The model under review builds one solid part; all positions refer to its coordinate system, in mm. A direction names the side the tool comes from. Coordinates: 2 decimals unless noted, no trailing zeros. Order: outer loops, then holes, each group sorted by start corner. A loop starts at its lowest first (then second) coordinate and runs counter-clockwise, first axis right, second up. Notation, with made-up numbers: (-39.75, 54) -> (-10.75, 54) arc R25 ccw to (-10.75, 68) -> close; hole circle Ø11 at (48, 25.5). An arc over 180 degrees is marked (long way). Use one line per item in the form item = value. Start each with the question number.
(1) Wall thickness on line 1 along X through (y, z) = (-2.4, 19); line 2 along X through (y, z) = (-2.5, -15.25); line 3 along Z through (x, y) = (-9.5, -0.75): over which ranges is each line inside the solid? List them lowest first.
(2) Insertion check: pin 1 Ø1.7 at (x, z) = (14.5, 14) entering from -Y; pin 2 Ø1 at (y, z) = (-1, -61.5) entering from +X. Each pin has a flat end and moves straight along its axis. Give the tip position at first contact, or say it passes through.
(3) Take a section at B-B (z = -50). State the section outline as (x, y) points.
(4) Mouldability with a two-part tool opening along X and no side actions: class faces 1 (the flat face through (-1, 0, -1)), 2 (the cylindrical face through (-39, -1, -50)), 3 (the flat face through (68.84, -1.48, 68.53)) as +X half, -X half, draft (parallel to the pull), parting line (faces both ways), or undercut.
(5) Take a section at C-C (y = -1.5). State how many separate pieces and enclosed holes the cut face has, then the cut area to 3 significant figures.
(6) For faces 4 (the cylindrical face through (-13.324, -2.507, -17.351)), 5 (the cylindrical face through (7, -1, -50)), 6 (the flat face through (-68.84, -1.48, -68.53)), list the 3-axis set-ups (+Z, -Z, +X, -X, +Y, -Y) from which the entire face can be reached by the end or side of a thin tool; tool diameter is ignored.
(7) Take a section at A-A (x = -26.5). State the section outline as (y, z) points, then the cut area to 3 significant figures.
```python
from build123d import *

# Parameters (mm, degrees)
SKETCH1_W                                  = 160
SKETCH1_H                                  = 160
BOSS_EXTRUDE1_DEPTH                        = 3
CUT_EXTRUDE2_REACH                         = 115.177
CUT_EXTRUDE1_REACH                         = 115.177
SKETCH2_R                                  = 2.55
MIRROR2_AT_THE_SECOND_PLANE_COPY_1_REACH   = 115.177
MIRROR2_AT_THE_SECOND_PLANE_COPY_2_REACH   = 115.177
MIRROR2_AT_THE_SECOND_PLANE_COPY_2_SKETC_R = 2.55
CUT_EXTRUDE3_REACH                         = 115.177
SKETCH8_R                                  = 1.525
CUT_EXTRUDE4_REACH                         = 115.177
SKETCH10_R                                 = 2.85
CUT_EXTRUDE6_DEPTH                         = 1


with BuildPart() as part:
    # Sketch1 → Boss-Extrude1 (new body)
    with BuildSketch(Plane(origin=(0, 0, 0), x_dir=(1, 0, 0), z_dir=(0, 1, 0))):
        Rectangle(SKETCH1_W, SKETCH1_H)
    extrude(amount=-BOSS_EXTRUDE1_DEPTH)

    # Sketch6 → Cut-Extrude2 (cut, up to next)
    with BuildSketch(Plane(origin=(0, 0, 0), x_dir=(1, 0, 0), z_dir=(0, 1, 0)), mode=Mode.PRIVATE) as cut_extrude2_sk1:
        Polygon((-80, -57.372583002), (-57.372583002, -80), (-80, -80), align=None)
    cut_extrude2_tool1 = extrude(cut_extrude2_sk1.sketch, amount=-CUT_EXTRUDE2_REACH, mode=Mode.PRIVATE) & part.part
    cut_extrude2 = cut_extrude2_tool1.solids().sort_by_distance((-72.457528, 0, 72.457528))[0]
    add(cut_extrude2, mode=Mode.SUBTRACT)

    # Sketch2 → Cut-Extrude1 (cut, up to next)
    with BuildSketch(Plane(origin=(0, 0, 0), x_dir=(1, 0, 0), z_dir=(0, 1, 0)), mode=Mode.PRIVATE) as cut_extrude1_sk1:
        with Locations(Location((-67.272077939, -55.95836944, 0), (0, 0, 270))):
            Circle(SKETCH2_R)
    cut_extrude1_tool1 = extrude(cut_extrude1_sk1.sketch, amount=-CUT_EXTRUDE1_REACH, mode=Mode.PRIVATE) & part.part
    # Sketch2 → Cut-Extrude1 (cut, up to next)
    with BuildSketch(Plane(origin=(0, 0, 0), x_dir=(1, 0, 0), z_dir=(0, 1, 0)), mode=Mode.PRIVATE) as cut_extrude1_sk2:
        with Locations(Location((-55.95836944, -67.272077939, 0), (0, 0, 270))):
            Circle(SKETCH2_R)
    cut_extrude1_tool2 = extrude(cut_extrude1_sk2.sketch, amount=-CUT_EXTRUDE1_REACH, mode=Mode.PRIVATE) & part.part
    cut_extrude1_1 = cut_extrude1_tool1.solids().sort_by_distance((-67.272078, 0, 55.958369))[0]
    add(cut_extrude1_1, mode=Mode.SUBTRACT)
    cut_extrude1_2 = cut_extrude1_tool2.solids().sort_by_distance((-55.958369, 0, 67.272078))[0]
    add(cut_extrude1_2, mode=Mode.SUBTRACT)
    cut_extrude1 = cut_extrude1_1 + cut_extrude1_2  # Cut-Extrude1 as one shape, for the pattern or mirror that repeats it

    # Mirror2: Cut-Extrude2, Cut-Extrude1 across plane
    add(cut_extrude2.mirror(Plane(origin=(0, 0, 0), x_dir=(0, 0, 1), z_dir=(1, 0, 0))), mode=Mode.SUBTRACT)
    add(cut_extrude1.mirror(Plane(origin=(0, 0, 0), x_dir=(0, 0, 1), z_dir=(1, 0, 0))), mode=Mode.SUBTRACT)

    # Mirror2 at the second plane: Cut-Extrude2, Cut-Extrude1 across plane
    add(cut_extrude2.mirror(Plane.XY), mode=Mode.SUBTRACT)
    add(cut_extrude1.mirror(Plane.XY), mode=Mode.SUBTRACT)

    # Mirror2 at the second plane copy 1 sketc → Mirror2 at the second plane copy 1 (cut, up to next)
    with BuildSketch(Plane(origin=(0, 0, 0), x_dir=(-1, 0, 0), z_dir=(0, 1, 0)), mode=Mode.PRIVATE) as mirror2_at_the_second_plane_copy_1_sk1:
        Polygon((-80, -57.372583002), (-57.372583002, -80), (-80, -80), align=None)
    mirror2_at_the_second_plane_copy_1_tool1 = extrude(mirror2_at_the_second_plane_copy_1_sk1.sketch, amount=-MIRROR2_AT_THE_SECOND_PLANE_COPY_1_REACH, mode=Mode.PRIVATE) & part.part
    add(mirror2_at_the_second_plane_copy_1_tool1.solids().sort_by_distance((72.457528, 0, -72.457528))[0], mode=Mode.SUBTRACT)

    # Mirror2 at the second plane copy 2 sketc → Mirror2 at the second plane copy 2 (cut, up to next)
    with BuildSketch(Plane(origin=(0, 0, 0), x_dir=(-1, 0, 0), z_dir=(0, 1, 0)), mode=Mode.PRIVATE) as mirror2_at_the_second_plane_copy_2_sk1:
        with Locations(Location((-67.272077939, -55.95836944, 0), (0, 0, 270))):
            Circle(MIRROR2_AT_THE_SECOND_PLANE_COPY_2_SKETC_R)
    mirror2_at_the_second_plane_copy_2_tool1 = extrude(mirror2_at_the_second_plane_copy_2_sk1.sketch, amount=-MIRROR2_AT_THE_SECOND_PLANE_COPY_2_REACH, mode=Mode.PRIVATE) & part.part
    # Mirror2 at the second plane copy 2 sketc → Mirror2 at the second plane copy 2 (cut, up to next)
    with BuildSketch(Plane(origin=(0, 0, 0), x_dir=(-1, 0, 0), z_dir=(0, 1, 0)), mode=Mode.PRIVATE) as mirror2_at_the_second_plane_copy_2_sk2:
        with Locations(Location((-55.95836944, -67.272077939, 0), (0, 0, 270))):
            Circle(MIRROR2_AT_THE_SECOND_PLANE_COPY_2_SKETC_R)
    mirror2_at_the_second_plane_copy_2_tool2 = extrude(mirror2_at_the_second_plane_copy_2_sk2.sketch, amount=-MIRROR2_AT_THE_SECOND_PLANE_COPY_2_REACH, mode=Mode.PRIVATE) & part.part
    add(mirror2_at_the_second_plane_copy_2_tool1.solids().sort_by_distance((67.272078, 0, -55.958369))[0], mode=Mode.SUBTRACT)
    add(mirror2_at_the_second_plane_copy_2_tool2.solids().sort_by_distance((55.958369, 0, -67.272078))[0], mode=Mode.SUBTRACT)

    # Sketch8 → Cut-Extrude3 (cut, up to next)
    with BuildSketch(Plane(origin=(0, 0, 0), x_dir=(1, 0, 0), z_dir=(0, 1, 0)), mode=Mode.PRIVATE) as cut_extrude3_sk1:
        with Locations(Location((-15.25, 15.25, 0), (0, 0, 270))):
            Circle(SKETCH8_R)
    cut_extrude3_tool1 = extrude(cut_extrude3_sk1.sketch, amount=-CUT_EXTRUDE3_REACH, mode=Mode.PRIVATE) & part.part
    # Sketch8 → Cut-Extrude3 (cut, up to next)
    with BuildSketch(Plane(origin=(0, 0, 0), x_dir=(1, 0, 0), z_dir=(0, 1, 0)), mode=Mode.PRIVATE) as cut_extrude3_sk2:
        with Locations(Location((-15.25, -15.25, 0), (0, 0, 270))):
            Circle(SKETCH8_R)
    cut_extrude3_tool2 = extrude(cut_extrude3_sk2.sketch, amount=-CUT_EXTRUDE3_REACH, mode=Mode.PRIVATE) & part.part
    # Sketch8 → Cut-Extrude3 (cut, up to next)
    with BuildSketch(Plane(origin=(0, 0, 0), x_dir=(1, 0, 0), z_dir=(0, 1, 0)), mode=Mode.PRIVATE) as cut_extrude3_sk3:
        with Locations(Location((15.25, -15.25, 0), (0, 0, 270))):
            Circle(SKETCH8_R)
    cut_extrude3_tool3 = extrude(cut_extrude3_sk3.sketch, amount=-CUT_EXTRUDE3_REACH, mode=Mode.PRIVATE) & part.part
    # Sketch8 → Cut-Extrude3 (cut, up to next)
    with BuildSketch(Plane(origin=(0, 0, 0), x_dir=(1, 0, 0), z_dir=(0, 1, 0)), mode=Mode.PRIVATE) as cut_extrude3_sk4:
        with Locations(Location((15.25, 15.25, 0), (0, 0, 270))):
            Circle(SKETCH8_R)
    cut_extrude3_tool4 = extrude(cut_extrude3_sk4.sketch, amount=-CUT_EXTRUDE3_REACH, mode=Mode.PRIVATE) & part.part
    add(cut_extrude3_tool1.solids().sort_by_distance((-15.25, 0, -15.25))[0], mode=Mode.SUBTRACT)
    add(cut_extrude3_tool2.solids().sort_by_distance((-15.25, 0, 15.25))[0], mode=Mode.SUBTRACT)
    add(cut_extrude3_tool3.solids().sort_by_distance((15.25, 0, 15.25))[0], mode=Mode.SUBTRACT)
    add(cut_extrude3_tool4.solids().sort_by_distance((15.25, 0, -15.25))[0], mode=Mode.SUBTRACT)

    # Sketch9 → Cut-Extrude4 (cut, up to next)
    with BuildSketch(Plane(origin=(0, 0, 0), x_dir=(1, 0, 0), z_dir=(0, 1, 0)), mode=Mode.PRIVATE) as cut_extrude4_sk1:
        with BuildLine():
            Line((-45, 38), (-45, 12))
            ThreePointArc((-45, 12), (-50, 7), (-55, 12))
            Line((-55, 12), (-55, 38))
            ThreePointArc((-55, 38), (-50, 43), (-45, 38))
        make_face()
    cut_extrude4_tool1 = extrude(cut_extrude4_sk1.sketch, amount=-CUT_EXTRUDE4_REACH, mode=Mode.PRIVATE) & part.part
    # Sketch9 → Cut-Extrude4 (cut, up to next)
    with BuildSketch(Plane(origin=(0, 0, 0), x_dir=(1, 0, 0), z_dir=(0, 1, 0)), mode=Mode.PRIVATE) as cut_extrude4_sk2:
        with BuildLine():
            Line((-45, -12), (-45, -38))
            ThreePointArc((-45, -38), (-50, -43), (-55, -38))
            Line((-55, -38), (-55, -12))
            ThreePointArc((-55, -12), (-50, -7), (-45, -12))
        make_face()
    cut_extrude4_tool2 = extrude(cut_extrude4_sk2.sketch, amount=-CUT_EXTRUDE4_REACH, mode=Mode.PRIVATE) & part.part
    # Sketch9 → Cut-Extrude4 (cut, up to next)
    with BuildSketch(Plane(origin=(0, 0, 0), x_dir=(1, 0, 0), z_dir=(0, 1, 0)), mode=Mode.PRIVATE) as cut_extrude4_sk3:
        with BuildLine():
            Line((-34, 55), (-12, 55))
            ThreePointArc((-12, 55), (-7, 50), (-12, 45))
            Line((-12, 45), (-34, 45))
            ThreePointArc((-34, 45), (-39, 50), (-34, 55))
        make_face()
    cut_extrude4_tool3 = extrude(cut_extrude4_sk3.sketch, amount=-CUT_EXTRUDE4_REACH, mode=Mode.PRIVATE) & part.part
    # Sketch9 → Cut-Extrude4 (cut, up to next)
    with BuildSketch(Plane(origin=(0, 0, 0), x_dir=(1, 0, 0), z_dir=(0, 1, 0)), mode=Mode.PRIVATE) as cut_extrude4_sk4:
        with BuildLine():
            Line((12, 55), (34, 55))
            ThreePointArc((34, 55), (39, 50), (34, 45))
            Line((34, 45), (12, 45))
            ThreePointArc((12, 45), (7, 50), (12, 55))
        make_face()
    cut_extrude4_tool4 = extrude(cut_extrude4_sk4.sketch, amount=-CUT_EXTRUDE4_REACH, mode=Mode.PRIVATE) & part.part
    cut_extrude4_1 = cut_extrude4_tool1.solids().sort_by_distance((-50, 0, -25))[0]
    add(cut_extrude4_1, mode=Mode.SUBTRACT)
    cut_extrude4_2 = cut_extrude4_tool2.solids().sort_by_distance((-50, 0, 25))[0]
    add(cut_extrude4_2, mode=Mode.SUBTRACT)
    cut_extrude4_3 = cut_extrude4_tool3.solids().sort_by_distance((-23, 0, -50))[0]
    add(cut_extrude4_3, mode=Mode.SUBTRACT)
    cut_extrude4_4 = cut_extrude4_tool4.solids().sort_by_distance((23, 0, -50))[0]
    add(cut_extrude4_4, mode=Mode.SUBTRACT)
    cut_extrude4 = cut_extrude4_1 + cut_extrude4_2 + cut_extrude4_3 + cut_extrude4_4  # Cut-Extrude4 as one shape, for the pattern or mirror that repeats it

    # Mirror3: Cut-Extrude4 across plane
    add(cut_extrude4.mirror(Plane.XY), mode=Mode.SUBTRACT)

    # Mirror3 at the second plane: Cut-Extrude4 across plane
    add(cut_extrude4.mirror(Plane(origin=(0, 0, 0), x_dir=(0, 0, 1), z_dir=(1, 0, 0))), mode=Mode.SUBTRACT)

    # Sketch10 → Cut-Extrude6 (cut)
    with BuildSketch(Plane(origin=(0, -3, 0), x_dir=(1, 0, 0), z_dir=(0, 1, 0))):
        with Locations(Location((-15.25, 15.25, 0), (0, 0, 270))):
            Circle(SKETCH10_R)
        with Locations(Location((15.25, 15.25, 0), (0, 0, 270))):
            Circle(SKETCH10_R)
        with Locations(Location((15.25, -15.25, 0), (0, 0, 270))):
            Circle(SKETCH10_R)
        with Locations(Location((-15.25, -15.25, 0), (0, 0, 270))):
            Circle(SKETCH10_R)
    extrude(amount=CUT_EXTRUDE6_DEPTH, mode=Mode.SUBTRACT)


solid = part.part
```
Findings:
q1.line_1 = -80 to -55, -45 to 45, 55 to 80
q1.line_2 = -80 to -55, -45 to -18.1, -12.4 to 12.4, 18.1 to 45, 55 to 80
q1.line_3 = -80 to -54.33, -45.67 to 45.67, 54.33 to 80
q2.pin_1 = -2
q2.pin_2 = 76.37
q3.outline = (-80, -3) -> (-39, -3) -> (-39, 0) -> (-80, 0) -> close; (-7, -3) -> (7, -3) -> (7, 0) -> (-7, 0) -> close; (39, -3) -> (80, -3) -> (80, 0) -> (39, 0) -> close
q4.face_1 = draft
q4.face_2 = undercut
q4.face_3 = +X half
q5.separate_pieces = 1
q5.enclosed_holes = 20
q5.area = 21,800 mm²
q6.face_4 = -Y
q6.face_5 = +Y, -Y
q6.face_6 = -Z, -X, +Y, -Y
q7.outline = (-3, -80) -> (0, -80) -> (0, -55) -> (-3, -55) -> close; (-3, -45) -> (0, -45) -> (0, 45) -> (-3, 45) -> close; (-3, 55) -> (0, 55) -> (0, 80) -> (-3, 80) -> close
q7.area = 420 mm²
